from build123d import *

# Parameters (mm, degrees)
SKETCH1_R           = 76.2
SKETCH1_R_2         = 3.175
BOSS_EXTRUDE1_DEPTH = 12.7
SKETCH2_R           = 3.175
CUT_EXTRUDE1_DEPTH  = 12.7
CIRPATTERN1_COUNT   = 6


with BuildPart() as part:
    # Sketch1 → Boss-Extrude1 (new body)
    with BuildSketch(Plane(origin=(0, 0, 0), x_dir=(1, 0, 0), z_dir=(0, 1, 0))):
        with Locations(Location((0, 0, 0), (0, 0, 270))):
            Circle(SKETCH1_R)
        with Locations(Location((0, -63.5, 0), (0, 0, 270))):
            Circle(SKETCH1_R_2, mode=Mode.SUBTRACT)
        with Locations(Location((0, 63.5, 0), (0, 0, 270))):
            Circle(SKETCH1_R_2, mode=Mode.SUBTRACT)
    extrude(amount=BOSS_EXTRUDE1_DEPTH)

    # Sketch2 → Cut-Extrude1 (cut)
    with BuildSketch(Plane(origin=(76.2, 0, 0), x_dir=(0, 0, -1), z_dir=(1, 0, 0))):
        with Locations((0, 6.35)):
            Circle(SKETCH2_R)
    cut_extrude1 = extrude(amount=-CUT_EXTRUDE1_DEPTH, mode=Mode.SUBTRACT)

    # CirPattern1: Cut-Extrude1 ×6 about axis
    cirpattern1_axis = Axis((0, 0, 0), (0, 1, 0))
    for i in range(1, CIRPATTERN1_COUNT):
        add(cut_extrude1.rotate(cirpattern1_axis, i * 360 / CIRPATTERN1_COUNT), mode=Mode.SUBTRACT)


solid = part.part
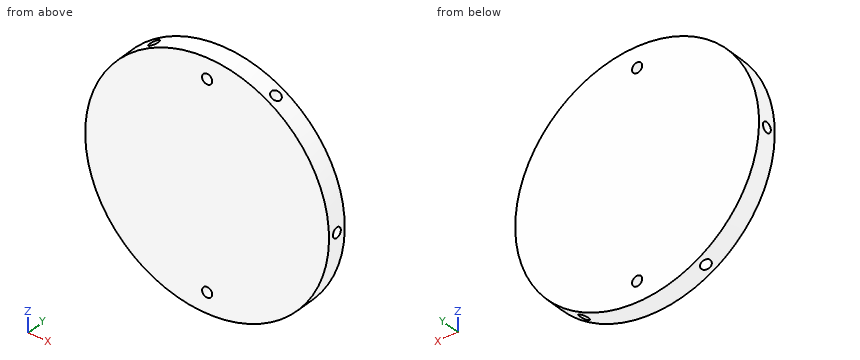
Could you check a few things on this model? Use its own coordinates, in mm. Coordinates: 2 decimals unless noted, no trailing zeros. Order: outer loops, then holes, each group sorted by start corner. A loop starts at its lowest first (then second) coordinate and runs counter-clockwise, first axis right, second up. Notation, with made-up numbers: (-17, 87) -> (20, 87) arc R23 ccw to (20, 123) -> close; hole circle Ø7 at (45, -26.75). An arc over 180 degrees is marked (long way). One line per item, written item: value. Start each with the question number.
1) Imagine slicing it at C-C on y = 6.35. List the corners of the cut face in (x, z) for me (3 decimals).
2) Imagine slicing it at B-B on x = 0. List the corners of the cut face in (y, z) for me (3 decimals), plus the area to 3 significant figures.
3) Imagine slicing it at D-D on x = -24.5. List the corners of the cut face in (y, z) for me, plus the area to 3 significant figures.
4) Imagine slicing it at A-A on z = 0. List the corners of the cut face in (x, y) for me (3 decimals), plus the area to 3 significant figures.
5) I'm going to push flat-ended pins straight in: pin 1 (4 mm diameter, centred on x = 0, z = -63.5, fed in from -Y); pin 2 (5 mm diameter, centred on y = 6, z = 1.5, fed in from -X); pin 3 (1.9 mm diameter, centred on y = 7, z = -1, fed in from +X); pin 4 (6 mm diameter, centred on y = 2.5, z = -56, fed in from -X). Where does each tip first touch, or does it pass through?
6) If I drill on L1, parallel to Z at x = -68.5, y = 8.75; L2, parallel to X at y = 7, z = -63.5 (3 decimals); L3, parallel to X at y = 6.25, z = 63.5 (3 decimals), over which ranges is the centre line in solid material (lowest first)? Write a range as [from, to].
Answer list:
1. outline: (-76.134, -3.175) arc R76.2 ccw to (-40.817, -64.346) -> (-34.5, -53.405) -> (-29, -56.58) -> (-35.317, -67.521) arc R76.2 ccw to (35.317, -67.521) -> (29, -56.58) -> (34.5, -53.405) -> (40.817, -64.346) arc R76.2 ccw to (76.134, -3.175) -> (63.5, -3.175) -> (63.5, 3.175) -> (76.134, 3.175) arc R76.2 ccw to (40.817, 64.346) -> (34.5, 53.405) -> (29, 56.58) -> (35.317, 67.521) arc R76.2 ccw to (-35.317, 67.521) -> (-29, 56.58) -> (-34.5, 53.405) -> (-40.817, 64.346) arc R76.2 ccw to (-76.134, 3.175) -> (-63.5, 3.175) -> (-63.5, -3.175) -> close; hole circle Ø6.35 at (0, -63.5); hole circle Ø6.35 at (0, 63.5)
2. outline: (0, -76.2) -> (12.7, -76.2) -> (12.7, -66.675) -> (0, -66.675) -> close; (0, -60.325) -> (12.7, -60.325) -> (12.7, 60.325) -> (0, 60.325) -> close; (0, 66.675) -> (12.7, 66.675) -> (12.7, 76.2) -> (0, 76.2) -> close
2. area: 1,770 mm2
3. outline: (0, -72.15) -> (12.7, -72.15) -> (12.7, 72.15) -> (0, 72.15) -> close
3. area: 1,830 mm2
4. outline: (-76.2, 0) -> (76.2, 0) -> (76.2, 3.175) -> (63.5, 3.175) -> (63.5, 9.525) -> (76.2, 9.525) -> (76.2, 12.7) -> (-76.2, 12.7) -> (-76.2, 9.525) -> (-63.5, 9.525) -> (-63.5, 3.175) -> (-76.2, 3.175) -> close
4. area: 1,770 mm2
5. pin 1: passes through
5. pin 2: stops at x = -76.19
5. pin 3: stops at x = 63.5
5. pin 4: stops at x = -54.75
6. L1: z = [-33.38, -2.08], [2.08, 33.38]
6. L2: x = [-42.121, -40.25], [-33.073, -3.175], [3.175, 33.073], [40.25, 42.121]
6. L3: x = [-42.121, -40.326], [-32.997, -3.175], [3.175, 32.997], [40.326, 42.121]
